The drawing under review shows one solid part. Ordinate dimensions are in mm from its lowest x, y, z. A direction names the side the tool comes from. Give positions to 0.01 mm unless a question says otherwise; leave off trailing zeros. Order: outer loops, then holes, each group sorted by start corner. A loop starts at its lowest first (then second) coordinate and runs counter-clockwise, first axis right, second up. Notation, with made-up numbers: (51, -22.5) -> (77, -22.5) arc R23 cw to (77, -7.5) -> close; hole circle Ø1 at (78.25, 48.25). An arc over 180 degrees is marked (long way). One line per item, written item: value. Start each with the question number.
1) For pin 1 (5.5 mm diameter, centred on x = 34.5, z = 9.5, fed in from +Y); pin 2 (8 mm diameter, centred on x = 49, y = 10, fed in from +Z); pin 3 (5 mm diameter, centred on x = 8.5, z = 11.5, fed in from -Y); pin 4 (4 mm diameter, centred on x = 14.5, z = 4.5, fed in from +Y), all flat-tipped, find the tip position at first contact; note any pin that passes through.
2) Wall thickness on line 1 along Z through (x, y) = (42.5, 18.5); line 2 along Y through (x, z) = (26.5, 6.75); line 3 along X through (y, z) = (6.5, 1) (1 decimal): over which ranges is each line inside the solid? List them lowest first. Write a range as from..to.
3) Consider section B-B (x = 48). State the section outline as (y, z) points.
4) Consider section A-A (y = 13.5). State the section outline as (x, z) points (1 decimal), plus the area to 3 significant figures.
5) Consider section C-C (y = 18.5). State the section outline as (x, z) points (1 decimal), plus the area to 3 significant figures.
6) Tool access review of the marked faces 1, 2 and 3: name each direction out of +Z, -Z, +X, -X, +Y, -Y from which nothing blocks a thin tool from reaching the whole face with its end or side.
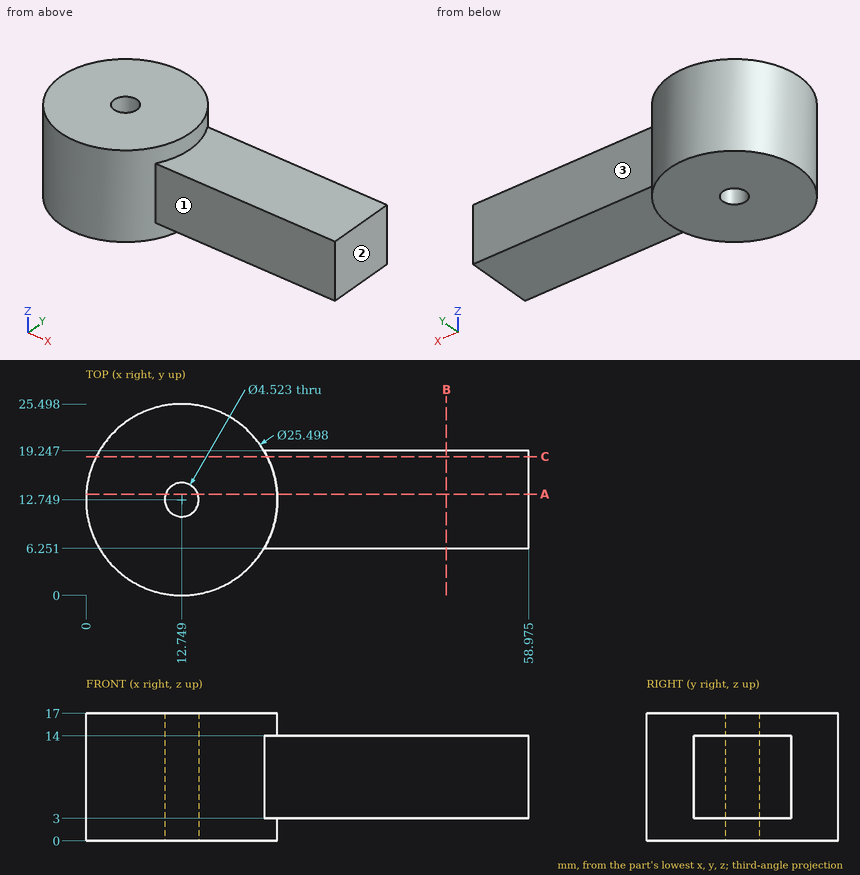
Checked values:
1. pin 1: stops at y = 19.25
1. pin 2: stops at z = 14
1. pin 3: stops at y = 0.12
1. pin 4: stops at y = 25.5
2. line 1: z = 3..14
2. line 2: y = 6.25..19.25
2. line 3: x = 1.6..23.9
3. outline: (6.25, 3) -> (19.25, 3) -> (19.25, 14) -> (6.25, 14) -> close
4. outline: (0, 0) -> (10.6, 0) -> (10.6, 17) -> (0, 17) -> close; (14.9, 0) -> (25.5, 0) -> (25.5, 3) -> (59, 3) -> (59, 14) -> (25.5, 14) -> (25.5, 17) -> (14.9, 17) -> close
4. area: 729 mm^2
5. outline: (1.4, 0) -> (24.1, 0) -> (24.1, 3) -> (59, 3) -> (59, 14) -> (24.1, 14) -> (24.1, 17) -> (1.4, 17) -> close
5. area: 770 mm^2
6. face 1: +Z, -Z, +X, -Y
6. face 2: +Z, -Z, +X, +Y, -Y
6. face 3: +Z, -Z, +X, +Y
